```python
from build123d import *

# Parameters (mm, degrees)
F1_DEPTH = 12.5
F0_W     = 3.5
F0_H     = 4.2426406871
F2_DEPTH = 18.5


with BuildPart() as f1:
    # F0 (on Top) → F1 (new body, symmetric)
    with BuildSketch(Plane.XY):
        with BuildLine():
            Line((-1.75, 2.1213203436), (1.75, 2.1213203436))
            ThreePointArc((1.75, 2.1213203436), (0, 2.75), (-1.75, 2.1213203436))
        make_face()
    extrude(amount=F1_DEPTH, both=True)



with BuildPart() as f1b:
    # F0 (on Top) → F1, piece 2 (new body, symmetric)
    with BuildSketch(Plane.XY):
        with BuildLine():
            ThreePointArc((-1.75, -2.1213203436), (0, -2.75), (1.75, -2.1213203436))
            Line((1.75, -2.1213203436), (-1.75, -2.1213203436))
        make_face()
    extrude(amount=F1_DEPTH, both=True)


with BuildPart() as f1_1:
    add(f1.part)

    add(f1b.part)  # F2 merges F1b
    # F0 (on Top) → F2 (join, symmetric)
    with BuildSketch(Plane.XY):
        Rectangle(F0_W, F0_H)
        with BuildLine():
            ThreePointArc((1.75, -2.1213203436), (2.4874685928, -1.17260394), (2.75, 0))
            ThreePointArc((2.75, 0), (2.4874685928, 1.17260394), (1.75, 2.1213203436))
            Line((1.75, 2.1213203436), (1.75, -2.1213203436))
        make_face()
        with BuildLine():
            Line((-1.75, -2.1213203436), (-1.75, 2.1213203436))
            ThreePointArc((-1.75, 2.1213203436), (-2.75, 0), (-1.75, -2.1213203436))
        make_face()
    extrude(amount=F2_DEPTH, both=True)


solid = f1_1.part
```
Part model, mm, in its own coordinate system. A direction names the side the tool comes from. Coordinates: 2 decimals unless noted, no trailing zeros. Order: outer loops, then holes, each group sorted by start corner. A loop starts at its lowest first (then second) coordinate and runs counter-clockwise, first axis right, second up. Notation, with made-up numbers: (-0.75, -14) - (10.25, -14) arc R12 ccw to (10.25, 2) - close; hole circle Ø1 at (80, 77.25). An arc over 180 degrees is marked (long way). Return JSON: item names as keys, results as strings. Group by question number.
Item 1: Pin check, flat tips, straight feed: pin 1 (0.5 mm diameter, centred on x = -1, y = 2.5, fed in from -Z); pin 2 (3 mm diameter, centred on x = 0, z = -15.5, fed in from -Y); pin 3 (2 mm diameter, centred on x = -2, z = 5, fed in from +Y); pin 4 (3 mm diameter, centred on y = -1, z = -0.5, fed in from -X). Stop position of each tip, or through.
Item 2: Cut at D-D (x = 1.3). List the corners of the cut face in (y, z).
Item 3: Cut at A-A (x = -1.1). List the corners of the cut face in (y, z), plus the area to 3 significant figures.
Item 4: Cut at B-B (z = -8.5). List the corners of the cut face in (x, y), plus the area to 3 significant figures.
Item 5: Which spindle directions (+Z, -Z, +X, -X, +Y, -Y) get a long thin tool onto all of the face, cutting with end or side? Do faces 1 (the face through (0, -2.121, 16)), 2 (the face through (0, -2.121, -15)), 3 (the face through (0, 2.121, -15)), 4 (the face through (0, 2.121, 16)). Say none if no direction does.
Item 6: Cut at C-C (y = -1.2). List the corners of the cut face in (x, z).
Item 7: Drill centre lines: probe 1 along Y at (x, z) = (0.2, -5); probe 2 along Z at (x, y) = (0.1, 2.35); probe 3 along Y at (x, z) = (1.6, -15). Where is each one in solid material? Low to high. Write a range as from..to.
Check values:
{
 "1": {"pin 1": "stops at z = -12.5", "pin 2": "stops at y = -2.12", "pin 3": "stops at y = 2.56", "pin 4": "stops at x = -2.75"},
 "2": {"outline": "(-2.42, -12.5) - (-2.12, -12.5) - (-2.12, -18.5) - (2.12, -18.5) - (2.12, -12.5) - (2.42, -12.5) - (2.42, 12.5) - (2.12, 12.5) - (2.12, 18.5) - (-2.12, 18.5) - (-2.12, 12.5) - (-2.42, 12.5) - close"},
 "3": {"outline": "(-2.52, -12.5) - (-2.12, -12.5) - (-2.12, -18.5) - (2.12, -18.5) - (2.12, -12.5) - (2.52, -12.5) - (2.52, 12.5) - (2.12, 12.5) - (2.12, 18.5) - (-2.12, 18.5) - (-2.12, 12.5) - (-2.52, 12.5) - close", "area": "177 mm2"},
 "4": {"outline": "circle Ø5.5 at (0, 0)", "area": "23.8 mm2"},
 "5": {"face 1": "+Z, +X, -X, -Y", "face 2": "-Z, +X, -X, -Y", "face 3": "-Z, +X, -X, +Y", "face 4": "+Z, +X, -X, +Y"},
 "6": {"outline": "(-2.47, -18.5) - (2.47, -18.5) - (2.47, 18.5) - (-2.47, 18.5) - close"},
 "7": {"probe 1": "y = -2.74..2.74", "probe 2": "z = -12.5..12.5", "probe 3": "y = -2.12..2.12"}
}
